from build123d import *

# Parameters (mm, degrees)
BOSS_EXTRUDE1_DEPTH = 20
SKETCH8_R           = 2.25
CUT_EXTRUDE3_DEPTH  = 5


with BuildPart() as part:
    # Sketch1 → Boss-Extrude1 (new body)
    with BuildSketch(Plane(origin=(0, 0, 0), x_dir=(1, 0, 0), z_dir=(0, 1, 0))):
        Polygon((0, 0), (46.42630295, -27.066325838), (36.746372501, 9.680088225), align=None)
    extrude(amount=-BOSS_EXTRUDE1_DEPTH)

    # Sketch8 → Cut-Extrude3 (cut)
    with BuildSketch(Plane(origin=(0, 0, 0), x_dir=(1, 0, 0), z_dir=(0, 1, 0))):
        with Locations(Location((20.085479714, -1.659955888, 0), (0, 0, 270))):
            Circle(SKETCH8_R)
        with Locations(Location((35.300766899, -10.348896383, 0), (0, 0, 270))):
            Circle(SKETCH8_R)
    extrude(amount=-CUT_EXTRUDE3_DEPTH, mode=Mode.SUBTRACT)


solid = part.part
Check sheet for the modelled part. Datum: model origin and axes. Units: mm. A direction names the side the tool comes from. Round coordinates to 2 decimals unless told otherwise and drop trailing zeros. Order: outer loops, then holes, each group sorted by start corner. A loop starts at its lowest first (then second) coordinate and runs counter-clockwise, first axis right, second up.
Q1. Cross-section at B-B, the plane y = -3.75. Enter the section's corners in (x, z).
Filled sheet:
outline: (0, 0) - (36.75, -9.68) - (46.43, 27.07) - close; hole circle Ø4.5 at (20.09, 1.66); hole circle Ø4.5 at (35.3, 10.35)
Q2. Set-up check for faces 5 (the face through (28, 0, 4)), 6 (the face through (37.532, -2.465, 10.056)): record each of +Z, -Z, +X, -X, +Y, -Y from which the full face is reachable in a straight line by a thin tool's end or side.
Filled sheet:
face 5: +Z, -Z, +X, -X, +Y
face 6: +Y
Q3. Cross-section at A-A, the plane z = 0.5. Enter the section's corners in (x, y).
Filled sheet:
outline: (0.86, -20) - (39.43, -20) - (39.43, 0) - (22.01, 0) - (22.01, -5) - (18.16, -5) - (18.16, 0) - (0.86, 0) - close
Q4. Scan lines: L1, parallel to X at y = -1.75, z = 8.5; L2, parallel to X at y = -6.25, z = 9; L3, parallel to Z at x = 26.5, y = -16.25. Record each from-to range of solid material in increasing order.
Filled sheet:
L1: x = 14.58 to 34.02, 36.58 to 41.54
L2: x = 15.44 to 41.67
L3: z = -6.98 to 15.45
Q5. Draft check along Z on faces 1 (the face through (41.654, -9.86, 8.95)), 2 (the face through (28, -20, 4)), 3 (the face through (20, -5, 2)), 4 (the face through (17.89, -2.46, 1.17)). Enter one of: pulls with the +Z half, pulls with the -Z half, needs draft (parallel to the pull), parting line crosses it, or undercut.
Filled sheet:
face 1: pulls with the -Z half
face 2: needs draft
face 3: undercut
face 4: undercut
Q6. Depth check by flat-ended pin: P1, Ø1, axis at x = 34.5, y = -14.5, coming from the +Z side; P2, Ø6, axis at x = 33.5, y = -9.5, coming from the +Z side; P3, Ø8, axis at y = -5, z = 18, coming from the +X side. Enter the tip coordinate at first touch or a pass-through.
Filled sheet:
P1: stops at z = 20.4
P2: stops at z = 21.28
P3: stops at x = 45.09
Q7. Cross-section at C-C, the plane y = -7. Enter the section's corners in (x, z).
Filled sheet:
outline: (0, 0) - (36.75, -9.68) - (46.43, 27.07) - close
Q8. Cross-section at D-D, the plane x = 30. Enter the section's corners in (y, z), plus the area to 3 significant figures.
Filled sheet:
outline: (-20, -7.9) - (0, -7.9) - (0, 17.49) - (-20, 17.49) - close
area: 508 mm2
